For this review, take the finished solid that the model builds, in its own axes (mm). A direction names the side the tool comes from. Coordinates: 2 decimals unless noted, no trailing zeros. Order: outer loops, then holes, each group sorted by start corner. A loop starts at its lowest first (then second) coordinate and runs counter-clockwise, first axis right, second up. Notation, with made-up numbers: (81, 13) - (88, 13) arc R25 cw to (88, 47) - close; hole circle Ø2 at (8, 58.25). An arc over 180 degrees is marked (long way). One line per item, written item: value. Start each with the question number.
(1) Clearance check with flat-ended pins moving along their axes: pin 1 (20 mm diameter, centred on x = -44, z = -28.5, fed in from +Y); pin 2 (5 mm diameter, centred on x = -16.5, z = 24, fed in from -Y); pin 3 (5 mm diameter, centred on y = -10.5, z = -24.5, fed in from +X). State where each tip first meets the part, or that it passes through.
(2) Consider section C-C on x = -35.5. Count the separate pieces of the cut face and the enclosed holes in it, then the cut area to 3 significant figures.
(3) Consider section D-D on y = -23. Write out the cut boundary in (x, z), then the cut area to 3 significant figures.
(4) Consider section B-B on z = 0. Write out the cut boundary in (x, y).
(5) For faces 1 (the flat face through (-35, -50, -30)), 2 (the flat face through (-36, -40, 21.5)), 3 (the flat face through (-36, -30, 19)), 4 (the flat face through (-32, -98, -28.5)), list the 3-axis set-ups (+Z, -Z, +X, -X, +Y, -Y) from which the entire face can be reached by the end or side of a thin tool; tool diameter is ignored.
(6) Consider section A-A on y = -108. Write out the cut boundary in (x, z).
(7) To check wall thickness, follow line 1 along Y through (x, z) = (-35, -31); line 2 along X through (y, z) = (-43.5, -26.5); line 3 along Y through (x, z) = (-35, 35). State the ranges of each line that lie inside material, in increasing order.
(8) Mouldability with a two-part tool opening along Z and no side actions: class faces 5 (the cylindrical face through (-35.86, -127.997, 35.556)), 6 (the flat face through (-36, -40, 16.5)), 7 (the flat face through (-35, -58, 0)), 8 (the cylindrical face through (-72.479, 0.66, 14.985)) as released by +Z, released by -Z, zero draft, split by the parting line, or undercut.
```python
from build123d import *

# Parameters (mm, degrees)
SKETCH1_R                 = 15
SKETCH1_W                 = 79
SKETCH1_H                 = 8
BOSS_EXTRUDE1_DEPTH       = 8
BOSS_EXTRUDE2_START       = 3
SKETCH1_3_R               = 15
SKETCH1_3_R_2             = 10
BOSS_EXTRUDE2_DEPTH       = 11
BOSS_EXTRUDE3_START       = -63
SKETCH1_4_R               = 15
SKETCH1_4_W               = 79
SKETCH1_4_H               = 8
BOSS_EXTRUDE3_DEPTH       = 8
LPATTERN3_COUNT           = 2
LPATTERN3_PITCH           = 66
SKETCH3_R                 = 15
SKETCH3_W                 = 63
SKETCH3_H                 = 8
SKETCH3_W_2               = 8
BOSS_EXTRUDE7_DEPTH       = 8
SKETCH3_7_R               = 15
SKETCH3_7_R_2             = 10
BOSS_EXTRUDE8_DEPTH       = 11
BOSS_EXTRUDE9_START       = -8
SKETCH4_R                 = 15
SKETCH4_W                 = 63
SKETCH4_H                 = 8
SKETCH4_W_2               = 8
BOSS_EXTRUDE9_DEPTH       = 8
BOSS_EXTRUDE10_START      = -11
SKETCH4_4_R               = 15
SKETCH4_4_R_2             = 10
BOSS_EXTRUDE10_DEPTH      = 11
SKETCH5_W                 = 55
SKETCH5_H                 = 8
SKETCH5_H_2               = 10
SKETCH5_H_3               = 33
SKETCH5_H_4               = 18
BOSS_EXTRUDE11_DEPTH      = 8
BOSS_EXTRUDE13_DEPTH      = 20
BOSS_EXTRUDE13_DEPTH_BACK = 8
SKETCH5_3_W               = 55
SKETCH5_3_H               = 5


with BuildPart() as part:
    # Sketch1 → Boss-Extrude1 (new body)
    # profile 1 of 2: a face of its own
    with BuildSketch(Plane(origin=(0, 0, 0), x_dir=(0, 0, -1), z_dir=(1, 0, 0))):
        with BuildLine():
            Line((39.5, -50), (18.791946309, 6.845637584))
            ThreePointArc((18.791946309, 6.845637584), (0, 20), (-18.791946309, 6.845637584))
            Line((-18.791946309, 6.845637584), (-39.5, -50))
            Line((-39.5, -50), (39.5, -50))
        make_face()
        Circle(SKETCH1_R, mode=Mode.SUBTRACT)
    # profile 2 of 2: a face of its own
    with BuildSketch(Plane(origin=(0, 0, 0), x_dir=(0, 0, -1), z_dir=(1, 0, 0))):
        with Locations((0, -54)):
            Rectangle(SKETCH1_W, SKETCH1_H)
    extrude(amount=-BOSS_EXTRUDE1_DEPTH)

    # Sketch1_3 → Boss-Extrude2 (add)
    with BuildSketch(Plane(origin=(0, 0, 0), x_dir=(0, 0, -1), z_dir=(1, 0, 0)).offset(BOSS_EXTRUDE2_START)):
        Circle(SKETCH1_3_R)
        Circle(SKETCH1_3_R_2, mode=Mode.SUBTRACT)
    boss_extrude2 = extrude(amount=-BOSS_EXTRUDE2_DEPTH)



with BuildPart() as body_2:
    # Sketch1_4 → Boss-Extrude3 (new body)
    # profile 1 of 2: a face of its own
    with BuildSketch(Plane(origin=(0, 0, 0), x_dir=(0, 0, -1), z_dir=(1, 0, 0)).offset(BOSS_EXTRUDE3_START)):
        with BuildLine():
            Line((39.5, -50), (18.791946309, 6.845637584))
            ThreePointArc((18.791946309, 6.845637584), (0, 20), (-18.791946309, 6.845637584))
            Line((-18.791946309, 6.845637584), (-39.5, -50))
            Line((-39.5, -50), (39.5, -50))
        make_face()
        Circle(SKETCH1_4_R, mode=Mode.SUBTRACT)
    # profile 2 of 2: a face of its own
    with BuildSketch(Plane(origin=(0, 0, 0), x_dir=(0, 0, -1), z_dir=(1, 0, 0)).offset(BOSS_EXTRUDE3_START)):
        with Locations((0, -54)):
            Rectangle(SKETCH1_4_W, SKETCH1_4_H)
    extrude(amount=-BOSS_EXTRUDE3_DEPTH)

    # LPattern3: Boss-Extrude2 ×2
    with Locations(*[(-i * LPATTERN3_PITCH, 0, 0) for i in range(1, LPATTERN3_COUNT)]):
        add(boss_extrude2)


with BuildPart() as part_1:
    add(part.part)

    add(body_2.part)  # Boss-Extrude7 merges body 2
    # Sketch3 → Boss-Extrude7 (add)
    # profile 1 of 3: a face of its own
    with BuildSketch(Plane.XY.offset(39.5)):
        with BuildLine():
            Line((-16.307748581, -113.626498508), (0, -58))
            Line((0, -58), (-63, -58))
            Line((-63, -58), (-71, -58))
            Line((-71, -58), (-54.692251419, -113.626498508))
            ThreePointArc((-54.692251419, -113.626498508), (-35.5, -128), (-16.307748581, -113.626498508))
        make_face()
        with Locations((-35.5, -108)):
            Circle(SKETCH3_R, mode=Mode.SUBTRACT)
    # profile 2 of 3: a face of its own
    with BuildSketch(Plane.XY.offset(39.5)):
        with Locations((-31.5, -54)):
            Rectangle(SKETCH3_W, SKETCH3_H)
    # profile 3 of 3: a face of its own
    with BuildSketch(Plane.XY.offset(39.5)):
        with Locations((-67, -54)):
            Rectangle(SKETCH3_W_2, SKETCH3_H)
    extrude(amount=-BOSS_EXTRUDE7_DEPTH)

    # Sketch3_7 → Boss-Extrude8 (add)
    with BuildSketch(Plane.XY.offset(39.5)):
        with Locations((-35.5, -108)):
            Circle(SKETCH3_7_R)
        with Locations((-35.5, -108)):
            Circle(SKETCH3_7_R_2, mode=Mode.SUBTRACT)
    extrude(amount=-BOSS_EXTRUDE8_DEPTH)

    # Sketch4 → Boss-Extrude9 (add)
    # profile 1 of 3: a face of its own
    with BuildSketch(Plane(origin=(0, 0, -39.5), x_dir=(-1, 0, 0), z_dir=(0, 0, -1)).offset(BOSS_EXTRUDE9_START)):
        with BuildLine():
            Line((54.692251419, -113.626498508), (71, -58))
            Line((71, -58), (8, -58))
            Line((8, -58), (0, -58))
            Line((0, -58), (16.307748581, -113.626498508))
            ThreePointArc((16.307748581, -113.626498508), (35.5, -128), (54.692251419, -113.626498508))
        make_face()
        with Locations(Location((35.5, -108, 0), (0, 0, 180))):
            Circle(SKETCH4_R, mode=Mode.SUBTRACT)
    # profile 2 of 3: a face of its own
    with BuildSketch(Plane(origin=(0, 0, -39.5), x_dir=(-1, 0, 0), z_dir=(0, 0, -1)).offset(BOSS_EXTRUDE9_START)):
        with Locations((39.5, -54)):
            Rectangle(SKETCH4_W, SKETCH4_H)
    # profile 3 of 3: a face of its own
    with BuildSketch(Plane(origin=(0, 0, -39.5), x_dir=(-1, 0, 0), z_dir=(0, 0, -1)).offset(BOSS_EXTRUDE9_START)):
        with Locations((4, -54)):
            Rectangle(SKETCH4_W_2, SKETCH4_H)
    extrude(amount=BOSS_EXTRUDE9_DEPTH)

    # Sketch4_4 → Boss-Extrude10 (add)
    with BuildSketch(Plane(origin=(0, 0, -39.5), x_dir=(-1, 0, 0), z_dir=(0, 0, -1)).offset(BOSS_EXTRUDE10_START)):
        with Locations(Location((35.5, -108, 0), (0, 0, 180))):
            Circle(SKETCH4_4_R)
        with Locations(Location((35.5, -108, 0), (0, 0, 180))):
            Circle(SKETCH4_4_R_2, mode=Mode.SUBTRACT)
    extrude(amount=BOSS_EXTRUDE10_DEPTH)

    # Sketch5 → Boss-Extrude11 (add)
    with BuildSketch(Plane(origin=(0, -50, 0), x_dir=(1, 0, 0), z_dir=(0, 1, 0))):
        with Locations((-35.5, -35.5)):
            Rectangle(SKETCH5_W, SKETCH5_H)
        with Locations((-35.5, -26.5)):
            Rectangle(SKETCH5_W, SKETCH5_H_2)
        with Locations((-35.5, 0)):
            Rectangle(SKETCH5_W, SKETCH5_H_3)
        with Locations((-35.5, 30.5)):
            Rectangle(SKETCH5_W, SKETCH5_H_4)
    extrude(amount=-BOSS_EXTRUDE11_DEPTH)

    # Sketch5_3 → Boss-Extrude13 (add, two sides: drawn at the far end of the back side and taken through both)
    with BuildSketch(Plane(origin=(0, -50, 0), x_dir=(1, 0, 0), z_dir=(0, 1, 0)).offset(-BOSS_EXTRUDE13_DEPTH_BACK)):
        with Locations((-35.5, 19)):
            Rectangle(SKETCH5_3_W, SKETCH5_3_H)
        with Locations((-35.5, -19)):
            Rectangle(SKETCH5_3_W, SKETCH5_3_H)
    extrude(amount=BOSS_EXTRUDE13_DEPTH + BOSS_EXTRUDE13_DEPTH_BACK)


solid = part_1.part
```
Geometry check:
1. pin 1: stops at y = -30
1. pin 2: stops at y = -58
1. pin 3: stops at x = 0
2. separate pieces: 3
2. enclosed holes: 0
2. area: 1,690 mm^2
3. outline: (-71, -29.66) - (-63, -29.66) - (-63, 29.66) - (-71, 29.66) - close; (-8, -29.66) - (0, -29.66) - (0, 29.66) - (-8, 29.66) - close
3. area: 949 mm^2
4. outline: (-74, -15) - (-71, -15) - (-71, -58) - (0, -58) - (0, -15) - (3, -15) - (3, -10) - (-8, -10) - (-8, -50) - (-63, -50) - (-63, -10) - (-74, -10) - close; (-74, 10) - (-63, 10) - (-63, 20) - (-71, 20) - (-71, 15) - (-74, 15) - close; (-8, 10) - (3, 10) - (3, 15) - (0, 15) - (0, 20) - (-8, 20) - close
5. face 1: -Z, +Y
5. face 2: +Z, +Y
5. face 3: +Z, -Z, +Y
5. face 4: +X, -X, -Y
6. outline: (-56.34, -39.5) - (-45.5, -39.5) - (-45.5, -28.5) - (-50.5, -28.5) - (-50.5, -31.5) - (-56.34, -31.5) - close; (-56.34, 31.5) - (-50.5, 31.5) - (-50.5, 28.5) - (-45.5, 28.5) - (-45.5, 39.5) - (-56.34, 39.5) - close; (-25.5, -39.5) - (-14.66, -39.5) - (-14.66, -31.5) - (-20.5, -31.5) - (-20.5, -28.5) - (-25.5, -28.5) - close; (-25.5, 28.5) - (-20.5, 28.5) - (-20.5, 31.5) - (-14.66, 31.5) - (-14.66, 39.5) - (-25.5, 39.5) - close
7. line 1: y = -122.99 to -117.99, -98.01 to -93.01, -58 to -50
7. line 2: x = -71 to -63, -8 to 0
7. line 3: y = -127.99 to -117.99, -98.01 to -50
8. face 5: zero draft
8. face 6: undercut
8. face 7: undercut
8. face 8: split by the parting line
